Autodesk Inventor part; units mm, degrees
ref_plane "YZ Plane" through (0, 0, 0) normal (1, 0, 0) x (0, 1, 0)
ref_plane "XZ Plane" through (0, 0, 0) normal (0, 1, 0) x (-1, 0, 0)
ref_plane "XY Plane" through (0, 0, 0) normal (0, 0, 1) x (1, 0, 0)
sketch "Sketch1" plane through (0, 0, 0) normal (0, 0, 1) x (1, 0, 0)
  line L0 (-12.7, 0) -> (12.7, 0)
  line L1 (-12.7, 0) -> (-12.7, 25.4)
  line L2 (12.7, 0) -> (12.7, 25.4)
  line L3 (-9.525, 25.4) -> (-9.525, 3.175)
  line L4 (-9.525, 3.175) -> (9.525, 3.175)
  line L5 (9.525, 3.175) -> (9.525, 25.4)
  line L6 (-12.7, 25.4) -> (-9.525, 25.4)
  line L7 (9.525, 25.4) -> (12.7, 25.4)
  point P0 (0, 0)
  point P1 (0, 0)
  dimension "d0" = 25.4
  dimension "d1" = 25.4
  dimension "d2" = 25.4
  dimension "d3" = 3.175
extrude "Extrusion1" add sketch "Sketch1" along normal mid plane 25.4
sketch "Sketch2" plane through (-9.525, 3.175, 12.7) normal (0, 1, 0) x (1, 0, 0)
  circle A0 centre (4.525, 17.7) radius 2
  circle A1 centre (4.525, 7.7) radius 2
  circle A2 centre (14.525, 7.7) radius 2
  circle A3 centre (14.525, 17.7) radius 2
  point P0 (9.525, 12.7)
  dimension "d6" = 4
  dimension "d7" = 5
  dimension "d8" = 5
  dimension "d11" = 360
hole "Hole1" at (-5, 3.175, 5) at (-5, 3.175, -5) at (5, 3.175, -5) at (5, 3.175, 5) direction (0, -1, 0) diameter 4 depth 3.175 countersink diameter 8 countersink angle 90
sketch "Sketch3" plane through (12.7, 0, 12.7) normal (1, 0, 0) x (0, 0, -1)
  line L0 (25.4, 3.175) -> (0, 3.175) construction
  line L1 (0, 25.4) -> (0, 3.175) construction
  line L2 (25.4, 25.4) -> (0, 25.4) construction
  line L3 (25.4, 3.175) -> (25.4, 25.4) construction
  line L4 (25.4, 25.4) -> (0, 25.4) construction
  line L5 (12.7, 25.4) -> (12.7, 3.175) construction
  circle A0 centre (6.7, 20.2875) radius 2
  circle A1 centre (6.7, 8.2875) radius 2
  circle A2 centre (18.7, 8.2875) radius 2
  circle A3 centre (18.7, 20.2875) radius 2
  line L6 (0, 14.2875) -> (25.4, 14.2875) construction
  point P0 (12.7, 0)
  point P1 (12.7, 14.2875)
  dimension "d20" = 4
  dimension "d21" = 6
  dimension "d22" = 6
  dimension "d25" = 360
extrude "Extrusion2" cut sketch "Sketch3" against normal through all
properties part number "Arashtrix 1in x 1in C-Bracket"
Verification items for the finished model (mm, model axes). Give positions to 0.01 mm unless a question says otherwise; leave off trailing zeros. Loops run counter-clockwise (first coordinate to the right, second up) from the corner with the lowest first, then second, coordinate; pieces in that order, holes last.
1. Section check A-A, the plane y = 4. Enter the section's corners in (x, z) (3 decimals).
2. Section check C-C, the plane y = 7. Enter the section's corners in (x, z) (3 decimals), then the cut area to 3 significant figures.
3. Section check B-B, the plane x = 5. Enter the section's corners in (y, z) (3 decimals), then the cut area to 3 significant figures.
4. Section check D-D, the plane z = 5. Count the separate pieces of the cut face and the enclosed holes in it, then the cut area to 3 significant figures.
5. Thickness scan on line 1 (X direction, y = 0.4, z = -5); line 2 (Y direction, x = -10.35, z = 6). Record the ranges inside material, lowest first.
6. Mould release check, pull along X, two halves, no side actions. Record for faces 1 (the flat face through (9.525, 14, 0)), 2 (the flat face through (-12.7, 13, 0)), 3 (the cylindrical face through (-11.09, 18.335, 6.434)), 4 (the flat face through (0, 3.175, 0)): released by +X, released by -X, zero draft, split by the parting line, or undercut.
7. Go/stop test with flat-tipped pins: pin 1 Ø4.5 at (x, z) = (-5, -5) entering from +Y (3 decimals); pin 2 Ø2.5 at (y, z) = (20.29, -6) entering from -X; pin 3 Ø6.5 at (x, z) = (5, -5) entering from +Y (3 decimals); pin 4 Ø1 at (x, z) = (5.5, 1) entering from +Y (3 decimals). Record where each tip stops, or that it passes through.
Geometry says:
1. outline: (-12.7, -12.7) - (-9.525, -12.7) - (-9.525, 12.7) - (-12.7, 12.7) - close; (9.525, -12.7) - (12.7, -12.7) - (12.7, 12.7) - (9.525, 12.7) - close
2. outline: (-12.7, -12.7) - (-9.525, -12.7) - (-9.525, -7.53) - (-12.7, -7.53) - close; (-12.7, -4.47) - (-9.525, -4.47) - (-9.525, 4.47) - (-12.7, 4.47) - close; (-12.7, 7.53) - (-9.525, 7.53) - (-9.525, 12.7) - (-12.7, 12.7) - close; (9.525, -12.7) - (12.7, -12.7) - (12.7, -7.53) - (9.525, -7.53) - close; (9.525, -4.47) - (12.7, -4.47) - (12.7, 4.47) - (9.525, 4.47) - close; (9.525, 7.53) - (12.7, 7.53) - (12.7, 12.7) - (9.525, 12.7) - close
2. area: 122 mm2
3. outline: (0, -12.7) - (3.175, -12.7) - (3.175, -9) - (1.175, -7) - (0, -7) - close; (0, -3) - (1.175, -3) - (3.175, -1) - (3.175, 1) - (1.175, 3) - (0, 3) - close; (0, 7) - (1.175, 7) - (3.175, 9) - (3.175, 12.7) - (0, 12.7) - close
3. area: 47.2 mm2
4. separate pieces: 7
4. enclosed holes: 0
4. area: 144 mm2
5. line 1: x = -12.7 to -7, -3 to 3, 7 to 12.7
5. line 2: y = 0 to 6.29, 10.29 to 18.29, 22.29 to 25.4
6. face 1: undercut
6. face 2: released by -X
6. face 3: zero draft
6. face 4: undercut
7. pin 1: stops at y = 1.425
7. pin 2: passes through
7. pin 3: stops at y = 2.425
7. pin 4: stops at y = 3.175
